Can you work these out from the model? Positions are in its coordinate system, mm. Give positions to 0.01 mm unless a question says otherwise; leave off trailing zeros. Loops run counter-clockwise (first coordinate to the right, second up) from the corner with the lowest first, then second, coordinate; pieces in that order, holes last. Notation, with made-up numbers: (70, 58) - (93, 58) arc R13 cw to (93, 67) - close; hole circle Ø5 at (-18.5, 67.5). An arc over 180 degrees is marked (long way). Answer in a Markdown table with one row per item.
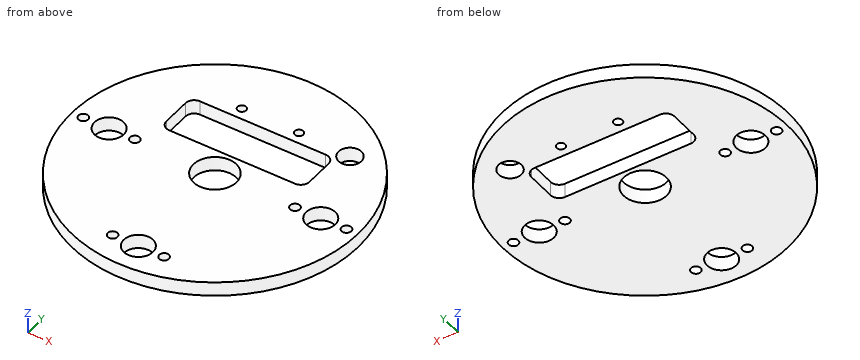
from build123d import *

# Parameters (mm, degrees)
SKETCH1_R                    = 50
BOSS_EXTRUDE1_DEPTH          = 5
F_15_0_15_DIAMETER_HOLE1_D   = 15
F_10_2_10_2_DIAMETER_HOLE1_D = 10.2
M3_CLEARANCE_HOLE1_D         = 3.4
CUT_EXTRUDE1_DEPTH           = 10
SKETCH10_R                   = 1.5
CUT_EXTRUDE2_DEPTH           = 10
SKETCH11_R                   = 4
CUT_EXTRUDE3_DEPTH           = 10


with BuildPart() as part:
    # Sketch1 → Boss-Extrude1 (new body)
    with BuildSketch(Plane.XY):
        Circle(SKETCH1_R)
    extrude(amount=BOSS_EXTRUDE1_DEPTH)

    # Ø15.0 (15) Diameter Hole1 (through all)
    with Locations(Plane(origin=(0, 0, 0), x_dir=(-1, 0, 0), z_dir=(0, 0, -1))):
        with Locations((0, 0)):
            Hole(F_15_0_15_DIAMETER_HOLE1_D / 2)

    # Ø10.2 (10.2) Diameter Hole1 (through all)
    with Locations(Plane(origin=(0, 0, 0), x_dir=(-1, 0, 0), z_dir=(0, 0, -1))):
        with Locations((37, 0), (-37, 0), (0, -40)):
            Hole(F_10_2_10_2_DIAMETER_HOLE1_D / 2)

    # M3 Clearance Hole1 (through all)
    with Locations(Plane.XY.offset(5)):
        with Locations((46, 0), (28, 0), (9, -40), (-9, -40), (-46, 0), (-28, 0)):
            Hole(M3_CLEARANCE_HOLE1_D / 2)

    # Sketch9 → Cut-Extrude1 (cut)
    with BuildSketch(Plane.XY.offset(5)):
        with BuildLine():
            Line((-22, 25), (22, 25))
            ThreePointArc((22, 25), (24.121320344, 24.121320344), (25, 22))
            Line((25, 22), (25, 12))
            ThreePointArc((25, 12), (24.121320344, 9.878679656), (22, 9))
            Line((22, 9), (-22, 9))
            ThreePointArc((-22, 9), (-24.121320344, 9.878679656), (-25, 12))
            Line((-25, 12), (-25, 22))
            ThreePointArc((-25, 22), (-24.121320344, 24.121320344), (-22, 25))
        make_face()
    extrude(amount=-CUT_EXTRUDE1_DEPTH, mode=Mode.SUBTRACT)

    # Sketch10 → Cut-Extrude2 (cut)
    with BuildSketch(Plane.XY.offset(5)):
        with Locations((-10, 29)):
            Circle(SKETCH10_R)
        with Locations((10, 29)):
            Circle(SKETCH10_R)
    extrude(amount=-CUT_EXTRUDE2_DEPTH, mode=Mode.SUBTRACT)

    # Sketch11 → Cut-Extrude3 (cut)
    with BuildSketch(Plane.XY.offset(5)):
        with Locations((28.284271247, 28.284271247)):
            Circle(SKETCH11_R)
    extrude(amount=-CUT_EXTRUDE3_DEPTH, mode=Mode.SUBTRACT)


solid = part.part
Q1. Imagine slicing it at A-A, the plane y = 0. Count the separate pieces of the cut face and the enclosed holes in it, and give its area (3 significant figures).
Checked values:
| item | result |
|---|---|
| separate pieces | 8 |
| enclosed holes | 0 |
| area | 255 mm² |
Q2. If I drill on line 1 (Y direction, x = 0, z = 1.4); line 2 (X direction, y = 15, z = 1.15); line 3 (Y direction, x = 6, z = 1.6), over which ranges is the centre line in solid material (lowest first)? Write a range as [from, to].
Checked values:
| item | result |
|---|---|
| line 1 | y = [-50, -45.1], [-34.9, -7.5], [7.5, 9], [25, 50] |
| line 2 | x = [-47.7, -25], [25, 47.7] |
| line 3 | y = [-49.64, -4.5], [4.5, 9], [25, 49.64] |
Q3. For pin 1 (1.5 mm diameter, centred on x = -37, z = 2, fed in from +Y), with a flat end and sliding along its axis, tell me the tip position at first contact or that it passes through.
Checked values:
| item | result |
|---|---|
| pin 1 | stops at y = 34.44 |
Q4. Imagine slicing it at C-C, the plane y = -40. Write out the boundary of the cut face in (x, z).
Checked values:
| item | result |
|---|---|
| outline | (-30, 0) - (-10.7, 0) - (-10.7, 5) - (-30, 5) - close; (-7.3, 0) - (-5.1, 0) - (-5.1, 5) - (-7.3, 5) - close; (5.1, 0) - (7.3, 0) - (7.3, 5) - (5.1, 5) - close; (10.7, 0) - (30, 0) - (30, 5) - (10.7, 5) - close |
Q5. Imagine slicing it at B-B, the plane x = 14. Write out the boundary of the cut face in (y, z).
Checked values:
| item | result |
|---|---|
| outline | (-48, 0) - (9, 0) - (9, 5) - (-48, 5) - close; (25, 0) - (48, 0) - (48, 5) - (25, 5) - close |
